from build123d import *

# Parameters (mm, degrees)
BOSS_EXTRUDE1_DEPTH      = 1
SKETCH1_3_W              = 2
SKETCH1_3_H              = 28
REVOLVE1_ANGLE           = 225
REVOLVE1_OTHER_WAY_ANGLE = 45


with BuildPart() as part:
    # Sketch1 → Boss-Extrude1 (new, symmetric)
    with BuildSketch(Plane(origin=(0, 0, 0), x_dir=(1, 0, 0), z_dir=(0, 1, 0))):
        Polygon((0, -30), (0, -29), (-3, -29), (-5, -29), (-5, -30), align=None)
        with BuildLine():
            ThreePointArc((0, -34), (-2, -32.000000008), (-1.7e-08, -30))
            Line((-1.7e-08, -30), (-5, -30))
            Line((-5, -30), (-5, -31))
            ThreePointArc((-5, -31), (-3.828427125, -33.828427125), (-1, -35))
            Line((-1, -35), (0, -35))
            Line((0, -35), (0, -34))
        make_face()
        Polygon((3, -29), (0, -29), (0, -30), (5, -30), (5, -29), align=None)
        with BuildLine():
            Line((5, -30), (-1.7e-08, -30))
            ThreePointArc((-1.7e-08, -30), (1.414213556, -30.585786432), (2, -32))
            ThreePointArc((2, -32), (1.414213562, -33.414213562), (0, -34))
            Line((0, -34), (0, -35))
            Line((0, -35), (1, -35))
            ThreePointArc((1, -35), (3.828427125, -33.828427125), (5, -31))
            Line((5, -31), (5, -30))
        make_face()
    extrude(amount=BOSS_EXTRUDE1_DEPTH, both=True)

    # Sketch1_3 → Revolve1 (revolve)
    with BuildSketch(Plane(origin=(0, 0, 0), x_dir=(1, 0, 0), z_dir=(0, 1, 0))):
        with Locations((-4, -15)):
            Rectangle(SKETCH1_3_W, SKETCH1_3_H)
        Polygon((0, -30), (0, -29), (-3, -29), (-5, -29), (-5, -30), align=None)
    revolve(axis=Axis((0, 0, 0), (0, 0, 1)), revolution_arc=REVOLVE1_ANGLE)

    # Sketch1_3 → Revolve1 other way (revolve)
    with BuildSketch(Plane(origin=(0, 0, 0), x_dir=(1, 0, 0), z_dir=(0, 1, 0))):
        with Locations((-4, -15)):
            Rectangle(SKETCH1_3_W, SKETCH1_3_H)
        Polygon((0, -30), (0, -29), (-3, -29), (-5, -29), (-5, -30), align=None)
    revolve(axis=Axis((0, 0, 0), (0, 0, -1)), revolution_arc=REVOLVE1_OTHER_WAY_ANGLE)


solid = part.part
Design review of the part built by this model. Coordinates are the model's own, in mm. A direction names the side the tool comes from. Round coordinates to 2 decimals unless told otherwise and drop trailing zeros. Write each loop counter-clockwise with the first axis right and the second up, starting at its lowest first coordinate (ties: lowest second). Pieces come first, ordered by that corner, then holes. Notation, with made-up numbers: (45, -12.5) - (72, -12.5) arc R26 cw to (72, 8.5) - close; hole circle Ø5 at (7.25, 59.5). An arc over 180 degrees is marked (long way). Use a Markdown table: item, result. Add a question column.
1. Wall thickness on probe 1 along Z at (x, y) = (0, 0.2); probe 2 along Z at (x, y) = (-4, 2.5); probe 3 along X at (y, z) = (-2.75, 19): over which ranges is each line inside the solid? List them lowest first.
2. We need section D-D (y = -1.75). State the section outline as (x, z) points, then the cut area to 3 significant figures.
3. We need section A-A (y = 1.75). State the section outline as (x, z) points, then the cut area to 3 significant figures.
4. For faces 1 (the face through (-3, 3, 15)), 2 (the face through (-3, 2, 30)), 3 (the face through (0, -3, 30)), 4 (the face through (0, 0, 29)), list the 3-axis set-ups (+Z, -Z, +X, -X, +Y, -Y) from which the entire face can be reached by the end or side of a thin tool; tool diameter is ignored.
5. Clearance check with flat-ended pins moving along their axes: pin 1 (5 mm diameter, centred on x = 4, z = 13, fed in from -Y); pin 2 (1.5 mm diameter, centred on x = -1, y = 1, fed in from -Z); pin 3 (3 mm diameter, centred on x = -0.5, y = -3, fed in from +Z); pin 4 (3.5 mm diameter, centred on x = 0, z = 32, fed in from +Y). State where each tip first meets the part, or that it passes through.
6. Mouldability with a two-part tool opening along X and no side actions: class faces 5 (the face through (0, 0, 34)), 6 (the face through (0, -4, 1)), 7 (the face through (-3.859, 0.014, 33.797)) as +X half, -X half, draft (parallel to the pull), parting line (faces both ways), or undercut.
7. We need section C-C (z = 32). State the section outline as (x, y) points, then the cut area to 3 significant figures.
8. We need section B-B (x = -0.5). State the section outline as (y, z) points, then the cut area to 3 significant figures.
Output:
| question | item | result |
|---|---|---|
| 1 | probe 1 | z = 29 to 30, 34 to 35 |
| 1 | probe 2 | z = 1 to 30 |
| 1 | probe 3 | x = -4.18 to -1.2, 1.2 to 4.18 |
| 2 | outline | (-4.68, 1) - (-2.44, 1) - (-2.44, 29) - (2.44, 29) - (2.44, 1) - (4.68, 1) - (4.68, 30) - (-4.68, 30) - close |
| 2 | area | 135 mm2 |
| 3 | outline | (-4.68, 1) - (-2.44, 1) - (-2.44, 29) - (-1.75, 29) - (-1.75, 30) - (-4.68, 30) - close; (1.75, 29) - (2.44, 29) - (2.44, 1) - (4.68, 1) - (4.68, 30) - (1.75, 30) - close |
| 3 | area | 132 mm2 |
| 4 | face 1 | +Z, -Z, +Y |
| 4 | face 2 | +Z, +X, -X, +Y |
| 4 | face 3 | +Z, +X, -X, -Y |
| 4 | face 4 | -Z |
| 5 | pin 1 | stops at y = -4.77 |
| 5 | pin 2 | stops at z = 29 |
| 5 | pin 3 | stops at z = 30 |
| 5 | pin 4 | passes through |
| 6 | face 5 | undercut |
| 6 | face 6 | draft |
| 6 | face 7 | -X half |
| 7 | outline | (-4.87, -1) - (-2, -1) - (-2, 1) - (-4.87, 1) - close; (2, -1) - (4.87, -1) - (4.87, 1) - (2, 1) - close |
| 7 | area | 11.5 mm2 |
| 8 | outline | (-4.97, 1) - (-2.96, 1) - (-2.96, 29) - (1, 29) - (1, 30.06) - (-1, 30.06) - (-1, 30) - (-4.97, 30) - close; (-1, 33.94) - (1, 33.94) - (1, 35) - (-1, 35) - close |
| 8 | area | 64.7 mm2 |
